Geometry check sheet. Reference: the model listing, model coordinates, mm. Face numbers are marked on the shaded views. Round coordinates to 2 decimals unless told otherwise and drop trailing zeros. Order: outer loops, then holes, each group sorted by start corner. A loop starts at its lowest first (then second) coordinate and runs counter-clockwise, first axis right, second up. Notation, with made-up numbers: (66.5, 72) - (116.5, 72) arc R25 cw to (116.5, 95) - close; hole circle Ø9 at (35.25, 21.25). An arc over 180 degrees is marked (long way). One line per question, with ' | ' between items. Start each with the question number.
Q1. Mould release check, pull along X, two halves, no side actions. Record for the marked faces 1, 2 and 3: +X half, -X half, draft (parallel to the pull), parting line (faces both ways), or undercut.
Q2. Sectioned sample at B-B, the plane x = 312. Enter the section's corners in (y, z).
Q3. Material ranges on line 1 along Y through (x, z) = (152, -0.75); line 2 along X through (y, z) = (5, -5.75); line 3 along Z through (x, y) = (250.5, -0.5), recorded low to high.
Q4. Gauge pin test, flat ends, axial feed: P1, Ø10, axis at x = 249.5, z = -0.5, coming from the -Y side; P2, Ø2, axis at x = 49, y = -3.5, coming from the +Z side; P3, Ø12, axis at x = 187, z = -4.5, coming from the +Y side. Record the tip position at first contact, or that the pin passes through.
Q5. Sectioned sample at A-A, the plane x = 53.5. Enter the section's corners in (y, z).
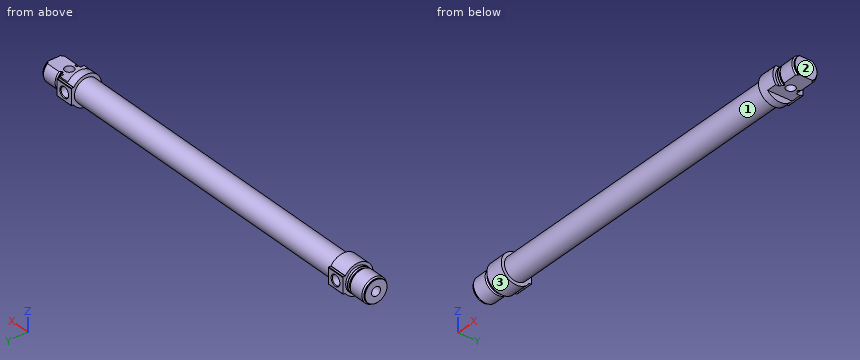
```python
from build123d import *

# Parameters (mm, degrees)
BOSS_EXTRUDE1_DEPTH     = 16
SKETCH3_W               = 286
SKETCH3_H               = 10.65
BOSS_EXTRUDE2_DEPTH     = 16
CUT_EXTRUDE1_DEPTH      = 13.5
CUT_EXTRUDE1_DEPTH_BACK = 13.5
HOLE1_D                 = 8
HOLE1_DEPTH             = 16
HOLE2_D                 = 8.566
HOLE2_DEPTH             = 13.5
HOLE2_CSINK_D           = 9.728
HOLE2_CSINK_ANGLE       = 90
HOLE3_D                 = 8.566
HOLE3_DEPTH             = 16
HOLE3_CSINK_D           = 9.728
HOLE3_CSINK_ANGLE       = 90
HOLE3_TIP               = 2.472791203


with BuildPart() as part:
    # Sketch1 → Revolve1 (revolve)
    with BuildSketch(Plane.XY):
        with BuildLine():
            Line((0, 0), (0, 9.8))
            Line((0, 9.8), (0.2, 10))
            Line((0.2, 10), (1, 10))
            Line((1, 10), (2, 11))
            Line((2, 11), (14.95, 11))
            Line((14.95, 11), (15.865685425, 10.084314575))
            ThreePointArc((15.865685425, 10.084314575), (16.125224104, 9.910896374), (16.43137085, 9.85))
            Line((16.43137085, 9.85), (17.2, 9.85))
            ThreePointArc((17.2, 9.85), (17.765685425, 10.084314575), (18, 10.65))
            Line((18, 10.65), (18, 11))
            Line((18, 11), (20, 11))
            Line((20, 11), (20, 0))
            Line((20, 0), (0, 0))
        make_face()
    revolve(axis=Axis((20, 0, 0), (-1, 0, 0)))

    # Sketch2 → Boss-Extrude1 (add)
    with BuildSketch(Plane(origin=(20, 0, 0), x_dir=(0, 0, -1), z_dir=(1, 0, 0))):
        with BuildLine():
            Line((7.25, 11.551515052), (7.25, 13.1))
            ThreePointArc((7.25, 13.1), (7.132842712, 13.382842712), (6.85, 13.5))
            Line((6.85, 13.5), (-6.85, 13.5))
            ThreePointArc((-6.85, 13.5), (-7.132842712, 13.382842712), (-7.25, 13.1))
            Line((-7.25, 13.1), (-7.25, 11.551515052))
            ThreePointArc((-7.25, 11.551515052), (-7.286144803, 11.408754992), (-7.385869565, 11.30039516))
            ThreePointArc((-7.385869565, 11.30039516), (0, -13.5), (7.385869565, 11.30039516))
            ThreePointArc((7.385869565, 11.30039516), (7.286144803, 11.408754992), (7.25, 11.551515052))
        make_face()
    extrude(amount=BOSS_EXTRUDE1_DEPTH)

    # Sketch3 → Revolve2 (revolve)
    with BuildSketch(Plane.XY):
        with Locations((179, 5.325)):
            Rectangle(SKETCH3_W, SKETCH3_H)
    revolve(axis=Axis((322, 0, 0), (-1, 0, 0)))

    # Sketch4 → Boss-Extrude2 (add)
    with BuildSketch(Plane(origin=(322, 0, 0), x_dir=(0, 0, -1), z_dir=(1, 0, 0))):
        with BuildLine():
            Line((7.25, 11.551515052), (7.25, 13.1))
            ThreePointArc((7.25, 13.1), (7.132842712, 13.382842712), (6.85, 13.5))
            Line((6.85, 13.5), (-6.85, 13.5))
            ThreePointArc((-6.85, 13.5), (-7.132842712, 13.382842712), (-7.25, 13.1))
            Line((-7.25, 13.1), (-7.25, 11.551515052))
            ThreePointArc((-7.25, 11.551515052), (-7.286144803, 11.408754992), (-7.385869565, 11.30039516))
            ThreePointArc((-7.385869565, 11.30039516), (0, -13.5), (7.385869565, 11.30039516))
            ThreePointArc((7.385869565, 11.30039516), (7.286144803, 11.408754992), (7.25, 11.551515052))
        make_face()
    extrude(amount=BOSS_EXTRUDE2_DEPTH)

    # Sketch5 → Revolve3 (revolve)
    with BuildSketch(Plane.XY):
        with BuildLine():
            Line((338, 0), (338, 11))
            Line((338, 11), (340, 11))
            Line((340, 11), (340, 10.65))
            ThreePointArc((340, 10.65), (340.234314575, 10.084314575), (340.8, 9.85))
            Line((340.8, 9.85), (341.56862915, 9.85))
            ThreePointArc((341.56862915, 9.85), (341.874775896, 9.910896374), (342.134314575, 10.084314575))
            Line((342.134314575, 10.084314575), (343.05, 11))
            Line((343.05, 11), (356, 11))
            Line((356, 11), (357, 10))
            Line((357, 10), (357.8, 10))
            Line((357.8, 10), (358, 9.8))
            Line((358, 9.8), (358, 0))
            Line((358, 0), (338, 0))
        make_face()
    revolve(axis=Axis((358, 0, 0), (-1, 0, 0)))

    # Sketch6 → Cut-Extrude1 (cut, two sides)
    with BuildSketch(Plane(origin=(0, 0, 0), x_dir=(1, 0, 0), z_dir=(0, 1, 0))) as cut_extrude1_sk:
        Polygon((329, 24), (329, 8), (358, 8), (358, -8), (329, -8), (329, -24), (374, -24), (374, 24), align=None)
    extrude(amount=CUT_EXTRUDE1_DEPTH, mode=Mode.SUBTRACT)
    extrude(cut_extrude1_sk.sketch, amount=-CUT_EXTRUDE1_DEPTH_BACK, mode=Mode.SUBTRACT)

    # Hole1
    with Locations(Plane(origin=(0, 0, -8), x_dir=(-1, 0, 0), z_dir=(0, 0, -1))):
        with Locations((-341, 0)):
            Hole(HOLE1_D / 2, depth=HOLE1_DEPTH)

    # Hole2
    with Locations(Plane(origin=(0, 13.5, 0), x_dir=(1, 0, 0), z_dir=(0, 1, 0))):
        with Locations((28.2, 0)):
            CounterSinkHole(HOLE2_D / 2, HOLE2_CSINK_D / 2, depth=HOLE2_DEPTH, counter_sink_angle=HOLE2_CSINK_ANGLE)

    # Hole3
    with Locations(Plane(origin=(0, 13.5, 0), x_dir=(1, 0, 0), z_dir=(0, 1, 0))):
        with Locations((329.8, 0)):
            CounterSinkHole(HOLE3_D / 2, HOLE3_CSINK_D / 2, depth=HOLE3_DEPTH, counter_sink_angle=HOLE3_CSINK_ANGLE)
            with Locations((0, 0, -(HOLE3_DEPTH + HOLE3_TIP / 2))):  # 120° drill point
                Cone(0, HOLE3_D / 2, HOLE3_TIP, mode=Mode.SUBTRACT)

    # Sketch13 → Cut-Revolve1 (revolve, cut)
    with BuildSketch(Plane.XY):
        Polygon((-4, 0), (-4, 4), (50.3, 4), (50.3, 10), (305.3, 10), (305.3, 0), align=None)
    revolve(axis=Axis((305.3, 0, 0), (-1, 0, 0)), mode=Mode.SUBTRACT)


solid = part.part
```
Determined:
1) face 1: undercut | face 2: +X half | face 3: draft
2) outline: circle Ø21.3 at (0, 0)
3) line 1: y = -10.62 to -9.97, 9.97 to 10.62 | line 2: x = 0 to 50.3, 305.3 to 358 | line 3: z = -10.64 to -9.99, 9.99 to 10.64
4) P1: stops at y = -10.65 | P2: stops at z = 10.35 | P3: stops at y = 10.65
5) outline: circle Ø21.3 at (0, 0); hole circle Ø20 at (0, 0)
